from build123d import *

# Parameters (mm, degrees)
SKETCH_1_W       = 225
SKETCH_1_H       = 200
SKETCH_1_R       = 90
EXTRUDE_1_DEPTH  = 2.5
SKETCH_9_W       = 225
SKETCH_9_H       = 120
EXTRUDE_11_DEPTH = 2.5
EXTRUDE_12_DEPTH = 2.5
EXTRUDE_13_DEPTH = 2.5
EXTRUDE_14_DEPTH = 2.5


with BuildPart() as part:
    # 草图1 → 凸台-拉伸1 (new body)
    with BuildSketch(Plane(origin=(0, 0, 0), x_dir=(1, 0, 0), z_dir=(0, 1, 0))):
        Rectangle(SKETCH_1_W, SKETCH_1_H)
        with Locations(Location((0, 0, 0), (0, 0, 270))):
            Circle(SKETCH_1_R, mode=Mode.SUBTRACT)
    extrude(amount=EXTRUDE_1_DEPTH)

    # 草图9 → 凸台-拉伸11 (add)
    with BuildSketch(Plane(origin=(0, -32.139380484, -88.302222156), x_dir=(1, 0, 0), z_dir=(0, 0.3420201433256658, 0.9396926207859095))):
        with Locations((0, 94.202014333)):
            Rectangle(SKETCH_9_W, SKETCH_9_H)
    extrude(amount=EXTRUDE_11_DEPTH)

    # 草图12 → 凸台-拉伸12 (add)
    with BuildSketch(Plane.ZY.offset(112.5)):
        Polygon((-100, 0), (-141.353630078, 113.618164853), (100, 113.618164853), (100, 0), align=None)
    extrude(amount=-EXTRUDE_12_DEPTH)

    # 草图13 → 凸台-拉伸13 (add)
    with BuildSketch(Plane(origin=(112.5, 0, 0), x_dir=(0, 0, -1), z_dir=(1, 0, 0))):
        Polygon((100, 0), (141.353630078, 113.618164853), (-100, 113.618164853), (-100, 0), align=None)
    extrude(amount=-EXTRUDE_13_DEPTH)

    # 草图15 → 凸台-拉伸14 (add)
    with BuildSketch(Plane.XY.offset(100)):
        Polygon((-112.5, 0), (-112.5, 113.791515023), (112.5, 113.618164853), (112.5, 0), align=None)
    extrude(amount=-EXTRUDE_14_DEPTH)


solid = part.part
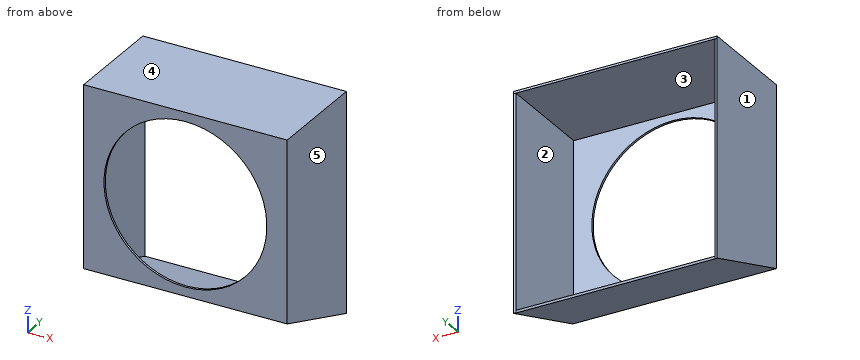
Build history of the part. All positions in model axes, mm. Face numbers are marked on the shaded views. A direction names the side the tool comes from. Give positions to 0.01 mm unless a question says otherwise; leave off trailing zeros. Loops run counter-clockwise (first coordinate to the right, second up) from the corner with the lowest first, then second, coordinate; pieces in that order, holes last. Notation, with made-up numbers: (38.5, 26) - (68.5, 26) arc R27 ccw to (68.5, 48) - close; hole circle Ø10 at (-38.5, -2). An arc over 180 degrees is marked (long way). Write item = value, one per line. Start each with the question number.
1) Drop flat-ended pins along their axis: pin 1 Ø2 at (x, z) = (-111.5, -52) entering from +Y; pin 2 Ø1.5 at (x, y) = (47.5, 13) entering from -Z. Give the stop position or say it passes through.
2) Pull direction Z, two halves, no side cores. Call the marked faces 3, 4 and 5: +Z half, -Z half, draft (parallel to the pull), parting line (faces both ways), or undercut.
3) Band-saw the part on A-A on z = 0. Give the cut face in (x, y), plus the area to 3 significant figures.
4) Band-saw the part on B-B on y = 14.5. Give the cut face in (x, z).
5) Band-saw the part on C-C on x = 63. Give the cut face in (y, z), plus the area to 3 significant figures.
6) Tool access for the marked faces 1 and 2: list every direction of +Z, -Z, +X, -X, +Y, -Y with a clear straight run to the whole face (end or side of a thin tool).
7) Probe probe 1 along X at (y, z) = (1.3, 0); probe 2 along X at (y, z) = (95.5, 45); probe 3 along Z at (x, y) = (-62.5, 92). List the from-to ranges inside material, lowest first. Write a range as from..to.
8) Band-saw the part on D-D on y = 97. Give the cut face in (x, z), plus the area to 3 significant figures.
Final values:
q1.pin_1 = 113.62
q1.pin_2 = -105
q2.face_3 = undercut
q2.face_4 = +Z half
q2.face_5 = draft
q3.outline = (-112.5, 0) - (-90, 0) - (-90, 2.5) - (-110, 2.5) - (-110, 113.62) - (-112.5, 113.62) - close; (90, 0) - (112.5, 0) - (112.5, 113.62) - (110, 113.62) - (110, 2.5) - (90, 2.5) - close
q3.area = 668 mm²
q4.outline = (-112.5, -105.28) - (112.5, -105.28) - (112.5, 100) - (-112.5, 100) - close; hole (-110, -102.62) - (110, -102.62) - (110, 97.5) - (-110, 97.5) - close
q5.outline = (0, -100) - (112.76, -141.04) - (113.62, -138.69) - (2.5, -98.25) - (2.5, -64.27) - (0, -64.27) - close; (0, 64.27) - (2.5, 64.27) - (2.5, 97.5) - (113.66, 97.5) - (113.66, 100) - (0, 100) - close
q5.area = 752 mm²
q6.face_1 = +Z, -Z, -X, +Y, -Y
q6.face_2 = +Y
q7.probe_1 = -112.5..-90, 90..112.5
q7.probe_2 = -112.5..-110, 110..112.5
q7.probe_3 = -133.49..-130.82, 97.5..100
q8.outline = (-112.5, -135.31) - (112.5, -135.31) - (112.5, 100) - (-112.5, 100) - close; hole (-110, -132.64) - (110, -132.64) - (110, 97.5) - (-110, 97.5) - close
q8.area = 2,310 mm²
